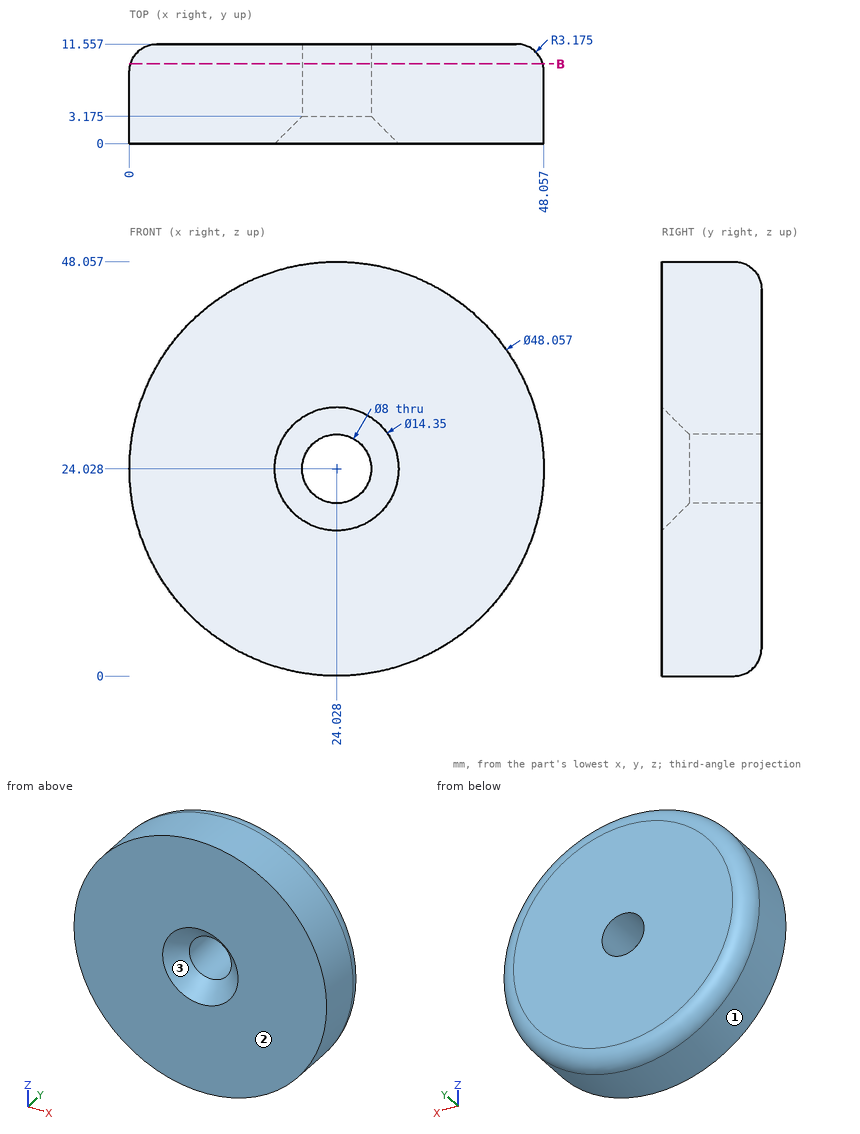
Part print with two shaded views. Sizes in mm from the minimum x, y, z corner. Round coordinates to 2 decimals unless told otherwise and drop trailing zeros. Order: outer loops, then holes, each group sorted by start corner. A loop starts at its lowest first (then second) coordinate and runs counter-clockwise, first axis right, second up. Notation, with made-up numbers: M 48.5,17 L 56.5,17 A21 ccw 56.5,46 Z; hole C -6.75,24.25 d7. An arc over 180 degrees is marked long. Use CSV: the item, a comma, the result in double quotes.
Item 1: Pin check, flat tips, straight feed: pin 1 (1.5 mm diameter, centred on x = 29.5, y = 9.5, fed in from -Z); pin 2 (13 mm diameter, centred on x = 24.03, z = 24.03, fed in from -Y); pin 3 (6 mm diameter, centred on x = 27.5, y = 6.5, fed in from -Z) (1 decimal). Stop position of each tip, or through.
Worked answers:
pin 1,"z = 0.57"
pin 2,"y = 0.67"
pin 3,"z = 0"
Item 2: Pull direction Z, two halves, no side cores. Call the marked faces 1, 2 and 3: released by +Z, released by -Z, zero draft, split by the parting line, or undercut.
Worked answers:
face 1,"split by the parting line"
face 2,"zero draft"
face 3,"undercut"
Item 3: Probe probe 1 along Y at (x, z) = (5, 33); probe 2 along Z at (x, y) = (24.5, 8) (1 decimal); probe 3 along X at (y, z) = (3.5, 22) (1 decimal). List the from-to ranges inside material, lowest first.
Worked answers:
probe 1,"0 to 11.55"
probe 2,"0 to 20.1, 28 to 48.1"
probe 3,"0.1 to 20.6, 27.5 to 48"
Item 4: Saw through at B-B (y = 9.25). List the corners of the cut face in (x, z) (1 decimal).
Worked answers:
outline,"C 24,24 d47.8; hole C 24,24 d8"
